Part model, mm, in its own coordinate system. Give positions to 0.01 mm unless a question says otherwise; leave off trailing zeros. Order: outer loops, then holes, each group sorted by start corner. A loop starts at its lowest first (then second) coordinate and runs counter-clockwise, first axis right, second up. Notation, with made-up numbers: (-1.5, 56) -> (35.5, 56) arc R29 ccw to (35.5, 83) -> close; hole circle Ø10 at (75, 84). An arc over 180 degrees is marked (long way). Write item = value, one per line. Start each with the question number.
(1) Saw through at C-C, the plane z = 6.5. State how many separate pieces and enclosed holes the cut face has, then the cut area to 3 significant figures.
(2) Flat gauge pins, fed straight in: pin 1 (1.5 mm diameter, centred on x = -88.5, z = 8.5, fed in from +Y); pin 2 (1 mm diameter, centred on y = -4.5, z = 6, fed in from -X); pin 3 (3 mm diameter, centred on y = -7, z = 2.5, fed in from -X); pin 4 (4 mm diameter, centred on x = 50, y = 11.5, fed in from -Z). Where does each tip first touch, or does it go through?
(3) Saw through at B-B, the plane y = 0. List the corners of the cut face in (x, z), then the cut area to 3 significant figures.
(4) Saw through at D-D, the plane x = 87. List the corners of the cut face in (y, z).
(5) Probe line 1 along Y through (x, z) = (-50, 7.25); line 2 along X through (y, z) = (21, 2.25); line 3 along X through (y, z) = (-23, 5). List the from-to ranges inside material, lowest first. Write a range as from..to.
(6) Saw through at A-A, the plane x = 210. List the corners of the cut face in (y, z).
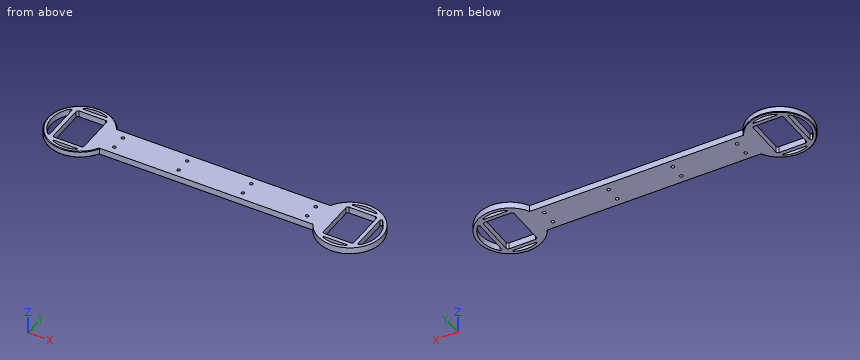
from build123d import *

# Parameters (mm, degrees)
SKETCH_1_W             = 47.4
SKETCH_1_H             = 66.4
SKETCH_1_R             = 2.5
EXTRUDE_1_DEPTH        = 10
FILLET_1_R             = 3
FILLET_2_R             = 2
FILLET_4_R             = 1
FILLET_5_R             = 1
FILLET_1_OF_MIRROR_1_R = 3
FILLET_2_OF_MIRROR_1_R = 2
FILLET_4_OF_MIRROR_1_R = 1


with BuildPart() as part:
    # 草图1 → 凸台-拉伸1 (new body)
    with BuildSketch(Plane.XY):
        with BuildLine():
            ThreePointArc((-165.866679255, 23.5), (-260, 0), (-165.866679255, -23.5))
            Line((-165.866679255, -23.5), (0, -23.5))
            Line((0, -23.5), (0, 23.5))
            Line((0, 23.5), (-165.866679255, 23.5))
        make_face()
        with BuildLine():
            ThreePointArc((-187.901131251, -39.2), (-210, -45), (-232.098868749, -39.2))
            Line((-232.098868749, -39.2), (-187.901131251, -39.2))
        make_face(mode=Mode.SUBTRACT)
        with BuildLine():
            ThreePointArc((-239.7, -33.806951948), (-255, 0), (-239.7, 33.806951948))
            Line((-239.7, 33.806951948), (-239.7, -33.806951948))
        make_face(mode=Mode.SUBTRACT)
        with Locations((-210, 0)):
            Rectangle(SKETCH_1_W, SKETCH_1_H, mode=Mode.SUBTRACT)
        with BuildLine():
            Line((-187.901131251, 39.2), (-232.098868749, 39.2))
            ThreePointArc((-232.098868749, 39.2), (-210, 45), (-187.901131251, 39.2))
        make_face(mode=Mode.SUBTRACT)
        with Locations((-50, 11.5)):
            Circle(SKETCH_1_R, mode=Mode.SUBTRACT)
        with Locations((-150, 11.5)):
            Circle(SKETCH_1_R, mode=Mode.SUBTRACT)
        with Locations((-150, -11.5)):
            Circle(SKETCH_1_R, mode=Mode.SUBTRACT)
        with Locations((-50, -11.5)):
            Circle(SKETCH_1_R, mode=Mode.SUBTRACT)
    extrude_1 = extrude(amount=EXTRUDE_1_DEPTH)

    # 圆角1
    fillet_1_edges = [part.edges().sort_by_distance(p)[0] for p in [
        (-186.3, 33.2, 5),
        (-233.7, 33.2, 5),
        (-233.7, -33.2, 5),
        (-186.3, -33.2, 5),
    ]]
    fillet(fillet_1_edges, radius=FILLET_1_R)

    # 圆角2
    fillet_2_edges = [part.edges().sort_by_distance(p)[0] for p in [
        (-239.7, 33.806951948, 5),
        (-239.7, -33.806951948, 5),
    ]]
    fillet(fillet_2_edges, radius=FILLET_2_R)

    # 圆角4
    fillet_4_edges = [part.edges().sort_by_distance(p)[0] for p in [
        (-187.901131251, 39.2, 5),
        (-232.098868749, 39.2, 5),
        (-187.901131251, -39.2, 5),
        (-232.098868749, -39.2, 5),
    ]]
    fillet(fillet_4_edges, radius=FILLET_4_R)

    # 圆角5
    fillet_5_edges = [part.edges().sort_by_distance(p)[0] for p in [
        (-260, 0, 10),
        (-260, 0, 0),
    ]]
    fillet(fillet_5_edges, radius=FILLET_5_R)

    # 镜向1: 凸台-拉伸1 across plane
    add(extrude_1.mirror(Plane(origin=(0, 0, 10), x_dir=(0, 0, 1), z_dir=(1, 0, 0))))

    # 圆角1 of 镜向1
    fillet_1_of_mirror_1_edges = [part.edges().sort_by_distance(p)[0] for p in [
        (186.3, 33.2, 5),
        (233.7, 33.2, 5),
        (233.7, -33.2, 5),
        (186.3, -33.2, 5),
    ]]
    fillet(fillet_1_of_mirror_1_edges, radius=FILLET_1_OF_MIRROR_1_R)

    # 圆角2 of 镜向1
    fillet_2_of_mirror_1_edges = [part.edges().sort_by_distance(p)[0] for p in [
        (239.7, 33.806951948, 5),
        (239.7, -33.806951948, 5),
    ]]
    fillet(fillet_2_of_mirror_1_edges, radius=FILLET_2_OF_MIRROR_1_R)

    # 圆角4 of 镜向1
    fillet_4_of_mirror_1_edges = [part.edges().sort_by_distance(p)[0] for p in [
        (187.901131251, 39.2, 5),
        (232.098868749, 39.2, 5),
        (187.901131251, -39.2, 5),
        (232.098868749, -39.2, 5),
    ]]
    fillet(fillet_4_of_mirror_1_edges, radius=FILLET_4_OF_MIRROR_1_R)


solid = part.part
Results list:
q1.separate_pieces = 1
q1.enclosed_holes = 16
q1.area = 22,400 mm^2
q2.pin_1 = 23.5
q2.pin_2 = -259.84
q2.pin_3 = -259.7
q2.pin_4 = through
q3.outline = (-260, 1) arc R1 ccw to (-259, 0) -> (-255, 0) -> (-255, 10) -> (-259, 10) arc R1 ccw to (-260, 9) -> close; (-239.7, 0) -> (-233.7, 0) -> (-233.7, 10) -> (-239.7, 10) -> close; (-186.3, 0) -> (186.3, 0) -> (186.3, 10) -> (-186.3, 10) -> close; (233.7, 0) -> (239.7, 0) -> (239.7, 10) -> (233.7, 10) -> close; (255, 0) -> (260, 0) -> (260, 10) -> (255, 10) -> close
q3.area = 3,950 mm^2
q4.outline = (-23.5, 0) -> (23.5, 0) -> (23.5, 10) -> (-23.5, 10) -> close
q5.line_1 = -23.5..-14, -9..9, 14..23.5
q5.line_2 = -255.38..-249.8, -239.7..-233.7, -186.3..186.3, 233.7..239.7, 249.8..255.38
q5.line_3 = -254.4..-248.68, -239.7..-233.7, -186.3..186.3, 233.7..239.7, 248.68..254.4
q6.outline = (-50, 0) -> (-45, 0) -> (-45, 10) -> (-50, 10) -> close; (-39.2, 0) -> (-33.2, 0) -> (-33.2, 10) -> (-39.2, 10) -> close; (33.2, 0) -> (39.2, 0) -> (39.2, 10) -> (33.2, 10) -> close; (45, 0) -> (50, 0) -> (50, 10) -> (45, 10) -> close
